Study the drawing (mm; zero at the part's minimum x, y, z) and answer. A direction names the side the tool comes from. Round coordinates to 2 decimals unless told otherwise and drop trailing zeros. Write each loop counter-clockwise with the first axis right and the second up, starting at its lowest first coordinate (ties: lowest second). Pieces come first, ordered by that corner, then holes.
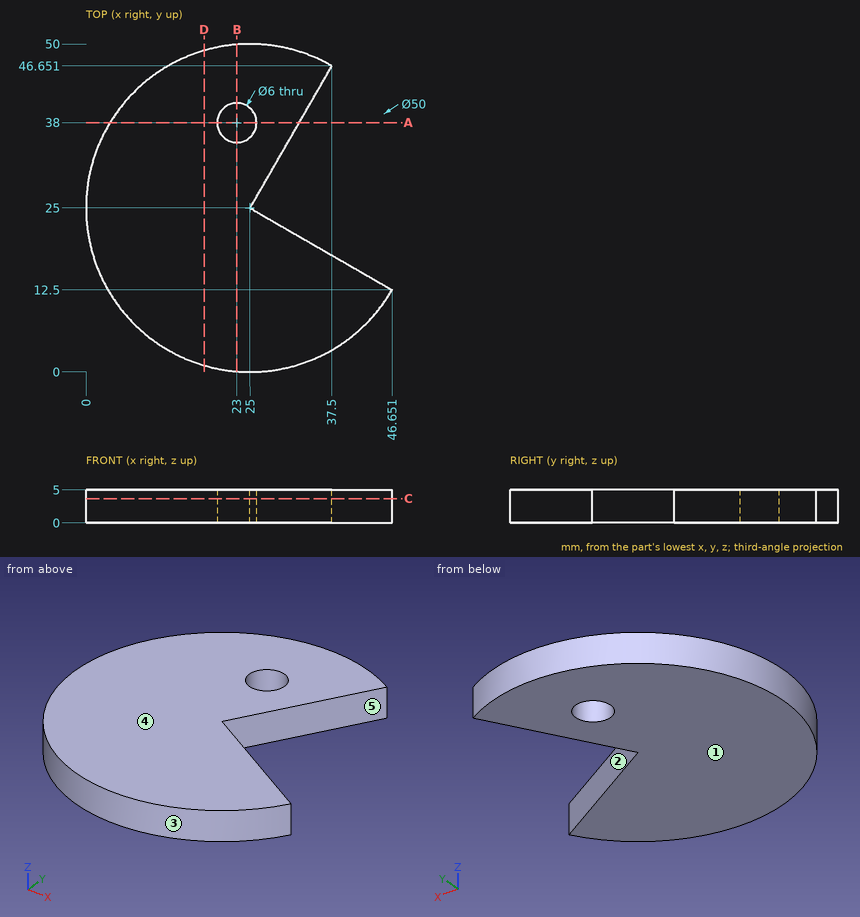
1. A tool of negligible diameter and unlimited length cuts with its end or side. For the marked faces 4 and 5, from which of +Z, -Z, +X, -X, +Y, -Y can it reach the whole face along a straight path? Write none if from no direction.
Geometry says:
face 4: +Z, +X, -X, +Y, -Y
face 5: +Z, -Z, +X
2. Section B-B on x = 23 is taken. Determine the outline of the cut face in (y, z).
Geometry says:
outline: (0.08, 0) - (35, 0) - (35, 5) - (0.08, 5) - close; (41, 0) - (49.92, 0) - (49.92, 5) - (41, 5) - close
3. Straight lines are drawn through the part: line 1 along Y through (x, z) = (25.5, 0.6) (1 decimal); line 2 along Y through (x, z) = (30.5, 2.45) (1 decimal); line 3 along Y through (x, z) = (23, 1.5). For each, find the intervals that lie inside material, in ascending order.
Geometry says:
line 1: y = 0 to 24.7, 25.9 to 36.3, 39.7 to 50
line 2: y = 0.6 to 21.8, 34.5 to 49.4
line 3: y = 0.08 to 35, 41 to 49.92
4. Section A-A on y = 38 is taken. Determine the outline of the cut face in (x, z) (1 decimal).
Geometry says:
outline: (3.6, 0) - (20, 0) - (20, 5) - (3.6, 5) - close; (26, 0) - (32.5, 0) - (32.5, 5) - (26, 5) - close
5. For a pull along Y with two mould halves and no side action, classify the marked faces 1, 2 and 3 as released by +Y, released by -Y, zero draft, split by the parting line, or undercut.
Geometry says:
face 1: zero draft
face 2: undercut
face 3: split by the parting line
6. Given pin 1 (1 mm diameter, centred on x = 33.5, z = 4, fed in from -Y) (1 decimal), flat-ended and moving along its own axis, determine where the tip first touches the part or whether it passes through.
Geometry says:
pin 1: stops at y = 1.3
7. Section D-D on x = 18 is taken. Determine the outline of the cut face in (y, z), plus the area to 3 significant figures.
Geometry says:
outline: (1, 0) - (49, 0) - (49, 5) - (1, 5) - close
area: 240 mm2
8. Section C-C on z = 3.7 is taken. Determine the outline of the cut face in (x, y), plus the area to 3 significant figures.
Geometry says:
outline: (25, 25) - (37.5, 46.65) arc R25 ccw (long way) to (46.65, 12.5) - close; hole circle Ø6 at (23, 38)
area: 1,440 mm2
